Autodesk Inventor part; units mm, degrees
ref_plane "YZ Plane" through (0, 0, 0) normal (1, 0, 0) x (0, 1, 0)
ref_plane "XZ Plane" through (0, 0, 0) normal (0, 1, 0) x (-1, 0, 0)
ref_plane "XY Plane" through (0, 0, 0) normal (0, 0, 1) x (1, 0, 0)
sketch "Sketch1" plane through (0, 0, 0) normal (0, 1, 0) x (-1, 0, 0)
  line L0 (37.9585, -11.217) -> (-26.0415, -11.217)
  line L1 (-26.0415, -11.217) -> (-26.0415, -107.217)
  line L2 (-26.0415, -107.217) -> (37.9585, -107.217)
  line L3 (37.9585, -107.217) -> (37.9585, -11.217)
  line L4 (13.9585, -107.217) -> (13.9585, -87.217)
  arc A0 (13.9585, -87.217) -> (-2.0415, -87.217) centre (5.9585, -87.217) ccw
  line L5 (-2.0415, -87.217) -> (-2.0415, -107.217)
  point P0 (0, 0)
  dimension "d0" = 64
  dimension "d1" = 96
  dimension "d2" = 20
  dimension "d3" = 8
  dimension "d4" = 32
extrude "Extrusion1" add sketch "Sketch1" along normal blind 16 contours L3 L2 L4 A0 L5 L1 L0
sketch "Sketch2" plane through (0, 16, 0) normal (0, 1, 0) x (1, 0, 0)
  line L0 (-37.9585, 11.1917) -> (26.0415, 11.1917)
  line L1 (26.0415, 11.1917) -> (26.0415, 27.1917)
  line L2 (26.0415, 27.1917) -> (-37.9585, 27.1917)
  line L3 (-37.9585, 27.1917) -> (-37.9585, 11.1917)
  line L4 (26.0415, 11.217) -> (26.0415, 107.217)
  line L5 (-37.9585, 107.217) -> (-37.9585, 11.217)
  point P0 (0, 0)
  dimension "d7" = 16
extrude "Extrusion2" add sketch "Sketch2" along normal blind 64
chamfer "Chamfer1" distance 20 distance2 30 1 edges at (26.0415, 80, -19.1917) measured on face at (4.7081, 80, -16.525)
sketch "Sketch4" plane through (-37.9585, 0, -107.217) normal (-1, 0, 0) x (0, 0, 1)
  line L0 (80.0253, 15.9344) -> (80.0253, 41.9344)
  line L1 (80.0253, 41.9344) -> (72.0253, 41.9344)
  arc A0 (48.0253, 41.9344) -> (72.0253, 41.9344) centre (60.0253, 41.9344) ccw
  line L2 (48.0253, 41.9344) -> (40.0253, 41.9344)
  line L3 (40.0253, 41.9344) -> (40.0253, 15.9344)
  line L4 (40.0253, 15.9344) -> (80.0253, 15.9344)
  line L5 (80.0253, 16) -> (80.0253, 80)
  point P0 (107.217, 0)
  dimension "d19" = 26
  dimension "d20" = 8
  dimension "d21" = 8
  dimension "d22" = 12
extrude "Extrusion4" add sketch "Sketch4" against normal blind 42
sketch "Sketch5" plane through (-37.9585, 0, -107.217) normal (-1, 0, 0) x (0, 0, 1)
  line L0 (40.044, 41.902) -> (0.0026, 15.8826)
  line L1 (0.0026, 15.8826) -> (40.044, 15.8826)
  line L2 (40.044, 15.8826) -> (40.044, 41.902)
  point P0 (107.217, 0)
extrude "Extrusion5" add sketch "Sketch5" against normal blind 12
equation "\"d4\" = 0.5 * d0"
properties part number "Exercise01"
Work out the finished part from the listing and answer in its coordinate system (mm). A direction names the side the tool comes from. Give positions to 0.01 mm unless a question says otherwise; leave off trailing zeros. Loops run counter-clockwise (first coordinate to the right, second up) from the corner with the lowest first, then second, coordinate; pieces in that order, holes last. Notation, with made-up numbers: (75.5, 31) -> (86.5, 31) arc R22 cw to (86.5, 44) -> close; hole circle Ø2 at (76, -18). An arc over 180 degrees is marked (long way). Put each result on its own line as item: value. Start each with the question number.
Item 1: The part is cut by section D-D (y = 28). Give the vertices of the cut face in (x, z).
Item 2: Which of the six approach directions +Z, -Z, +X, -X, +Y, -Y give full straight-line access (tool end or side, diameter ignored) to faces 4 (the face through (-17, 41.934, -63)), 5 (the face through (-6, 48, -11.192)), 6 (the face through (-13, 29, -67.192))?
Item 3: The part is cut by section C-C (z = -25.5). Give the vertices of the cut face in (x, y), then the cut area to 3 significant figures.
Item 4: The part is cut by section B-B (z = -100). Give the vertices of the cut face in (x, y).
Item 5: Find the intervals of material crossed by L1, parallel to Z at x = -26, y = 60; L2, parallel to Y at x = 20.5, z = -54; L3, parallel to Y at x = -30, z = -34.5, in increasing order. Write a range as [from, to].
Item 6: Each of these flat-tipped pins is pushed along its axis until it touches: P1, Ø20.5, axis at x = -23.5, y = 24.5, coming from the -Z side; P2, Ø6.5, axis at x = -19.5, z = -63, coming from the +Y side; P3, Ø20.5, axis at y = 30.5, z = -87.5, coming from the +X side; P4, Ø8, axis at y = 55.5, z = -23.5, coming from the +X side. Where does it stop, or does it pass through?
Item 7: The mould has two halves that part along X. Classify faces 1 (the face through (-16, 80, -19)), 2 (the face through (-25.958, 23, -79)), 3 (the face through (2.042, 8, -97)): released by +X, released by -X, zero draft, split by the parting line, or undercut.
Answers below:
1. outline: (-37.96, -88.57) -> (-25.96, -88.57) -> (-25.96, -67.19) -> (4.04, -67.19) -> (4.04, -27.19) -> (26.04, -27.19) -> (26.04, -11.19) -> (-37.96, -11.19) -> close
2. face 4: -Z, +X, -X, +Y
2. face 5: +Z, +X, -X, +Y, -Y
2. face 6: -Z, +X, +Y
3. outline: (-37.96, 0) -> (26.04, 0) -> (26.04, 50) -> (6.04, 80) -> (-37.96, 80) -> close
3. area: 4,820 mm2
4. outline: (-37.96, 0) -> (-13.96, 0) -> (-13.96, 16) -> (-25.96, 16) -> (-25.96, 20.57) -> (-37.96, 20.57) -> close; (2.04, 0) -> (26.04, 0) -> (26.04, 16) -> (2.04, 16) -> close
5. L1: [-27.19, -11.19]
5. L2: [0, 16]
5. L3: [0, 41.93]
6. P1: z = -107.22
6. P2: y = 41.93
6. P3: x = -25.96
6. P4: x = 25.04
7. face 1: zero draft
7. face 2: released by +X
7. face 3: undercut
